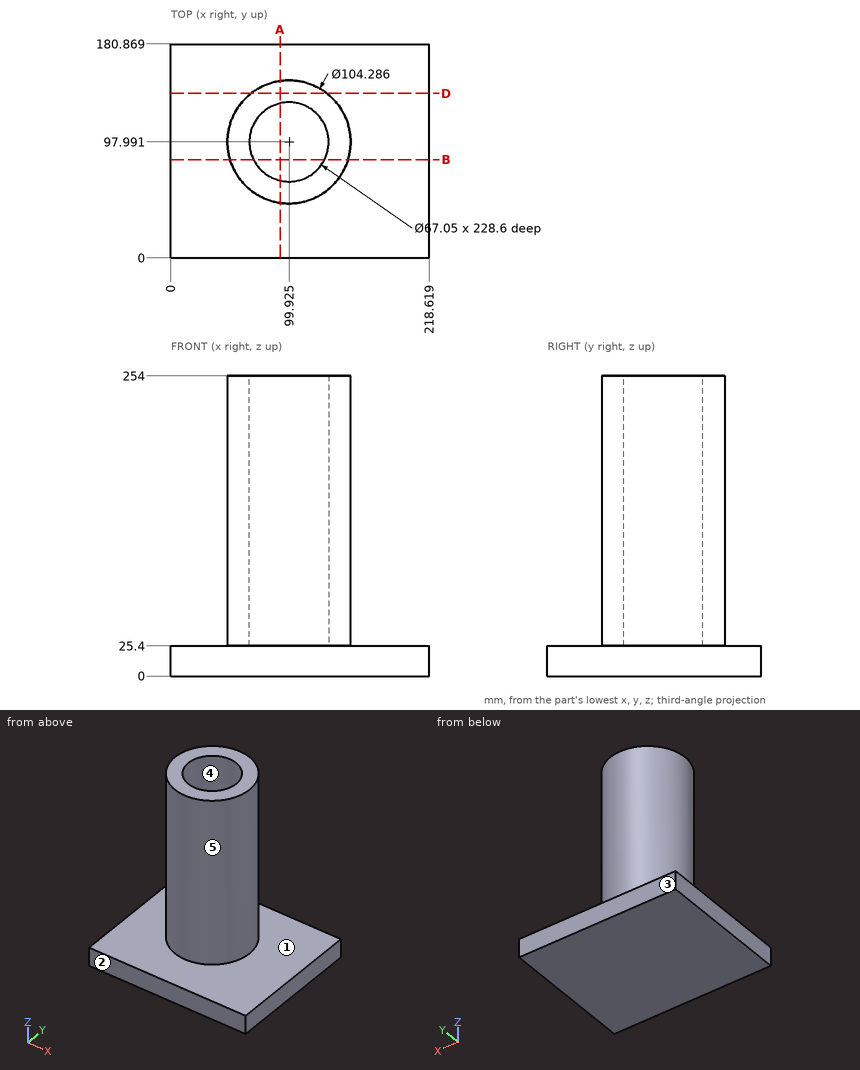
Job drawing, mm, ordinate dimensions from the low corner. One solid piece. A direction names the side the tool comes from. Coordinates: 2 decimals unless noted, no trailing zeros. Order: outer loops, then holes, each group sorted by start corner. A loop starts at its lowest first (then second) coordinate and runs counter-clockwise, first axis right, second up. Notation, with made-up numbers: (77.5, 57.25) - (119.5, 57.25) arc R18 ccw to (119.5, 86.25) - close; hole circle Ø6 at (34, 63). An arc over 180 degrees is marked (long way). Return JSON: item names as keys, results as strings. Group by question number.
1) Saw through at B-B, the plane y = 83. Write the cut outline in (x, z).
2) Flat gauge pins, fed straight in: P1, Ø5, axis at y = 118, z = 39, coming from the -X side; P2, Ø2, axis at x = 40, y = 112.5, coming from the -Z side; P3, Ø1, axis at x = 122.5, y = 161.5, coming from the +Z side; P4, Ø5, axis at y = 79, z = 29.5, coming from the +X side. Where does each tip first touch, or does it go through?
3) Saw through at A-A, the plane x = 92.5. Write the cut outline in (y, z).
4) Mould opens along X. For the marked faces 3, 4 and 5 say: released by +X, released by -X, zero draft, split by the parting line, or undercut.
5) Probe line 1 (Z direction, x = 82, y = 172); line 2 (Y direction, x = 100, z = 85.5); line 3 (Y direction, x = 78.5, z = 197.5) (1 decimal). List the from-to ranges inside material, lowest first. Write a range as from..to.
6) Saw through at D-D, the plane y = 139. Write the cut outline in (x, z), plus the area to 3 significant figures.
7) Tool access for the marked faces 1 and 2: list every direction of +Z, -Z, +X, -X, +Y, -Y with a clear straight run to the whole face (end or side of a thin tool).
Values found:
{
 "1": {"outline": "(0, 0) - (218.62, 0) - (218.62, 25.4) - (149.87, 25.4) - (149.87, 254) - (129.91, 254) - (129.91, 25.4) - (69.94, 25.4) - (69.94, 254) - (49.98, 254) - (49.98, 25.4) - (0, 25.4) - close"},
 "2": {"P1": "stops at x = 50.81", "P2": "stops at z = 0", "P3": "stops at z = 25.4", "P4": "stops at x = 149.39"},
 "3": {"outline": "(0, 0) - (180.87, 0) - (180.87, 25.4) - (149.6, 25.4) - (149.6, 254) - (130.68, 254) - (130.68, 25.4) - (65.3, 25.4) - (65.3, 254) - (46.38, 254) - (46.38, 25.4) - (0, 25.4) - close"},
 "4": {"face 3": "zero draft", "face 4": "undercut", "face 5": "split by the parting line"},
 "5": {"line 1": "z = 0..25.4", "line 2": "y = 45.85..64.47, 131.52..150.13", "line 3": "y = 50.5..72.2, 123.8..145.5"},
 "6": {"outline": "(0, 0) - (218.62, 0) - (218.62, 25.4) - (132.13, 25.4) - (132.13, 254) - (67.72, 254) - (67.72, 25.4) - (0, 25.4) - close", "area": "20,300 mm²"},
 "7": {"face 1": "+Z", "face 2": "+Z, -Z, +X, -X, -Y"}
}
